from build123d import *

# Parameters (mm, degrees)
SKETCH_1_R          = 1.5
SKETCH_1_R_2        = 1.75
EXTRUDE_1_DEPTH     = 9
FILLET_1_R          = 5
CUT_EXTRUDE_1_DEPTH = 3.5
SKETCH_5_R          = 3.1
CUT_EXTRUDE_2_DEPTH = 5
FILLET_2_R          = 0.5


with BuildPart() as part:
    # 草图1 → 凸台-拉伸1 (new body)
    with BuildSketch(Plane.XY):
        Polygon((27.354279807, 0), (-27.354279807, 0), (-53.690131677, -7.056670241), (-49.721245605, -21.868754713), (-47.133055154, -31.528012976), (-43.164169081, -46.340097448), (-33.746392275, -43.816611758), (-40.303468798, -19.345269023), (-26.283171214, -15.588541608), (-19.72609469, -40.059884343), (-16.828317211, -39.283427207), (16.828317211, -39.283427207), (19.72609469, -40.059884343), (26.283171214, -15.588541608), (40.303468798, -19.345269023), (33.746392275, -43.816611758), (43.164169081, -46.340097448), (47.133055154, -31.528012976), (49.721245605, -21.868754713), (53.690131677, -7.056670241), align=None)
        with Locations((-39.784585925, -35.770653663)):
            Circle(SKETCH_1_R, mode=Mode.SUBTRACT)
        with Locations((-17.863593392, -35.419723902)):
            Circle(SKETCH_1_R_2, mode=Mode.SUBTRACT)
        with Locations((17.863593392, -35.419723902)):
            Circle(SKETCH_1_R_2, mode=Mode.SUBTRACT)
        with Locations((39.784585925, -35.770653663)):
            Circle(SKETCH_1_R, mode=Mode.SUBTRACT)
        with Locations((-45.478604918, -14.520285484)):
            Circle(SKETCH_1_R, mode=Mode.SUBTRACT)
        with Locations((-22.347153069, -19.710269626)):
            Circle(SKETCH_1_R, mode=Mode.SUBTRACT)
        with Locations((-26.282483038, -4)):
            Circle(SKETCH_1_R_2, mode=Mode.SUBTRACT)
        with Locations((22.347153069, -19.710269626)):
            Circle(SKETCH_1_R, mode=Mode.SUBTRACT)
        with Locations((45.478604918, -14.520285484)):
            Circle(SKETCH_1_R, mode=Mode.SUBTRACT)
        with Locations((26.282483038, -4)):
            Circle(SKETCH_1_R_2, mode=Mode.SUBTRACT)
    extrude(amount=EXTRUDE_1_DEPTH)

    # 圆角1
    fillet_1_edges = [part.edges().sort_by_distance(p)[0] for p in [
        (16.828317211, -39.283427207, 4.5),
        (-16.828317211, -39.283427207, 4.5),
        (-43.164169081, -46.340097448, 4.5),
        (-53.690131677, -7.056670241, 4.5),
        (-27.354279807, 0, 4.5),
        (27.354279807, 0, 4.5),
        (53.690131677, -7.056670241, 4.5),
        (43.164169081, -46.340097448, 4.5),
    ]]
    fillet(fillet_1_edges, radius=FILLET_1_R)

    # 草图2 → 切除-拉伸1 (cut)
    with BuildSketch(Plane(origin=(0, 0, 0), x_dir=(-1, 0, 0), z_dir=(0, 0, -1))):
        Polygon((-42.411378471, -15.342146334), (-43.23323932, -12.274919887), (-46.300465767, -11.453059037), (-48.545831365, -13.698424635), (-47.723970515, -16.765651082), (-44.656744068, -17.587511931), align=None)
        Polygon((-21.52529222, -22.777496073), (-19.279926622, -20.532130476), (-20.101787472, -17.464904029), (-23.169013919, -16.643043179), (-25.414379516, -18.888408777), (-24.592518667, -21.955635224), align=None)
        Polygon((-36.717359478, -36.592514512), (-37.539220328, -33.525288065), (-40.606446775, -32.703427216), (-42.851812372, -34.948792813), (-42.029951523, -38.01601926), (-38.962725076, -38.83788011), align=None)
        Polygon((38.962725076, -38.83788011), (36.717359478, -36.592514512), (37.539220328, -33.525288065), (40.606446775, -32.703427216), (42.851812372, -34.948792813), (42.029951523, -38.01601926), align=None)
        Polygon((24.592518667, -21.955635224), (21.52529222, -22.777496073), (19.279926622, -20.532130476), (20.101787472, -17.464904029), (23.169013919, -16.643043179), (25.414379516, -18.888408777), align=None)
        Polygon((44.656744068, -17.587511931), (42.411378471, -15.342146334), (43.23323932, -12.274919887), (46.300465767, -11.453059037), (48.545831365, -13.698424635), (47.723970515, -16.765651082), align=None)
    extrude(amount=-CUT_EXTRUDE_1_DEPTH, mode=Mode.SUBTRACT)

    # 草图5 → 切除-拉伸2 (cut)
    with BuildSketch(Plane.XY.offset(9)):
        with Locations((-26.282483038, -4)):
            Circle(SKETCH_5_R)
        with Locations((-17.863593392, -35.419723902)):
            Circle(SKETCH_5_R)
        with Locations((17.863593392, -35.419723902)):
            Circle(SKETCH_5_R)
        with Locations((26.282483038, -4)):
            Circle(SKETCH_5_R)
    extrude(amount=-CUT_EXTRUDE_2_DEPTH, mode=Mode.SUBTRACT)

    # 圆角2
    fillet_2_edges = [part.edges().sort_by_distance(p)[0] for p in [
        (-20.963515007, -35.44176885, 6.5),
        (-20.559226734, -36.950593225, 6.5),
        (20.963515007, -35.44176885, 6.5),
        (20.559226734, -36.950593225, 6.5),
        (19.72609469, -40.059884343, 4.5),
        (-19.72609469, -40.059884343, 4.5),
        (-26.283171214, -15.588541608, 4.5),
        (-40.303468798, -19.345269023, 4.5),
        (-33.746392275, -43.816611758, 4.5),
        (33.746392275, -43.816611758, 4.5),
        (40.303468798, -19.345269023, 4.5),
        (26.283171214, -15.588541608, 4.5),
    ]]
    fillet(fillet_2_edges, radius=FILLET_2_R)


solid = part.part
Check sheet for the modelled part. Datum: model origin and axes. Units: mm. A direction names the side the tool comes from. Give positions to 0.01 mm unless a question says otherwise; leave off trailing zeros. Order: outer loops, then holes, each group sorted by start corner. A loop starts at its lowest first (then second) coordinate and runs counter-clockwise, first axis right, second up. Notation, with made-up numbers: M 52,-11 L 75,-11 A19 ccw 75,6 Z; hole C -18.75,30.25 d8. An arc over 180 degrees is marked long. Answer as CSV lines item,"result". Start each with the question number.
Item 1: Tool access check on faces 1 (the face through (18.34, -39.69, 4.44)), 2 (the face through (-41, -34, 3.5)), 3 (the face through (20, -35, 4)). Record the directions out of +Z, -Z, +X, -X, +Y, -Y that give a thin tool (end or side, any length) a straight path to the whole face; none if there is none.
Item 2: Thickness scan on line 1 (X direction, y = -29, z = 5.75); line 2 (Y direction, x = 10, z = 5.5); line 3 (X direction, y = -37.5, z = 1.25). Record the ranges inside material, lowest first. Write a range as [from, to].
Item 3: Cross-section at D-D on z = 5.5. State how many separate pieces and enclosed holes the cut face has, plus the area to 3 significant figures.
Item 4: Cross-section at C-C on y = -25. Enter the section's corners in (x, z), plus the area to 3 significant figures.
Item 5: Gauge pin test, flat ends, axial feed: P1, Ø6.5, axis at x = -23.5, y = -19.5, coming from the -Z side; P2, Ø4, axis at y = -38.5, z = 4.5, coming from the -X side; P3, Ø3, axis at x = 22.5, y = -19.5, coming from the -Z side; P4, Ø1.5, axis at y = -39.5, z = 2.5, coming from the +X side. Record the tip position at first contact, or that the pin passes through.
Item 6: Cross-section at B-B on x = -9.5. Enter the section's corners in (y, z).
Item 7: Mould release check, pull along X, two halves, no side actions. Record for faces 4 (the face through (47.41, -12.56, 1.73)), 5 (the face through (44.75, -11.87, 1.73)): +X half, -X half, draft (parallel to the pull), parting line (faces both ways), or undercut.
Item 8: Cross-section at A-A on y = -4. Enter the section's corners in (x, z).
Established:
1,face 1,"+Z, -Z, -Y"
1,face 2,"-Z"
1,face 3,"+Z"
2,line 1,"x = [-47.81, -37.72], [-22.69, 22.69], [37.72, 47.81]"
2,line 2,"y = [-39.28, 0]"
2,line 3,"x = [-45.53, -42.17], [-37.62, -35.44], [-20.41, 20.41], [35.44, 37.62], [42.17, 45.53]"
3,separate pieces,"1"
3,enclosed holes,"8"
3,area,"3,030 mm^2"
4,outline,"M -48.88,0 L -38.79,0 L -38.79,9 L -48.88,9 Z; M -23.76,0 L 23.76,0 L 23.76,9 L -23.76,9 Z; M 38.79,0 L 48.88,0 L 48.88,9 L 38.79,9 Z"
4,area,"609 mm^2"
5,P1,"stops at z = 0"
5,P2,"stops at x = -45.8"
5,P3,"stops at z = 3.5"
5,P4,"stops at x = 45.2"
6,outline,"M -39.28,0 L 0,0 L 0,9 L -39.28,9 Z"
7,face 4,"undercut"
7,face 5,"undercut"
8,outline,"M -42.28,0 L -28.03,0 L -28.03,4 L -29.38,4 L -29.38,9 L -42.28,9 Z; M -24.53,0 L 24.53,0 L 24.53,4 L 23.18,4 L 23.18,9 L -23.18,9 L -23.18,4 L -24.53,4 Z; M 28.03,0 L 42.28,0 L 42.28,9 L 29.38,9 L 29.38,4 L 28.03,4 Z"
